from build123d import *

# Parameters (mm, degrees)
F1_DEPTH = 25.4
F0_W     = 244.054224
F0_H     = 73.369068
F2_DEPTH = 23.283333
F3_DEPTH = 4.7625


with BuildPart() as f1:
    # F0 (on Front) → F1 (new body)
    with BuildSketch(Plane.XZ):
        with BuildLine():
            Line((137.143306, 54.800729), (-137.143306, 54.800729))
            ThreePointArc((-137.143306, 54.800729), (-139.264627, 53.922049), (-140.143306, 51.800729))
            Line((-140.143306, 51.800729), (-140.143306, -51.800729))
            ThreePointArc((-140.143306, -51.800729), (-139.264627, -53.922049), (-137.143306, -54.800729))
            Line((-137.143306, -54.800729), (137.143306, -54.800729))
            ThreePointArc((137.143306, -54.800729), (139.264627, -53.922049), (140.143306, -51.800729))
            Line((140.143306, -51.800729), (140.143306, 51.800729))
            ThreePointArc((140.143306, 51.800729), (139.264627, 53.922049), (137.143306, 54.800729))
        make_face()
        with BuildLine():
            ThreePointArc((-127.443306, 39.100729), (-126.564627, 41.222049), (-124.443306, 42.100729))
            Line((-124.443306, 42.100729), (124.443306, 42.100729))
            ThreePointArc((124.443306, 42.100729), (126.564627, 41.222049), (127.443306, 39.100729))
            Line((127.443306, 39.100729), (127.443306, -39.100729))
            ThreePointArc((127.443306, -39.100729), (126.564627, -41.222049), (124.443306, -42.100729))
            Line((124.443306, -42.100729), (-124.443306, -42.100729))
            ThreePointArc((-124.443306, -42.100729), (-126.564627, -41.222049), (-127.443306, -39.100729))
            Line((-127.443306, -39.100729), (-127.443306, 39.100729))
        make_face(mode=Mode.SUBTRACT)
    extrude(amount=F1_DEPTH)

    # F0 (on Front) → F2 (join)
    with BuildSketch(Plane.XZ):
        with BuildLine():
            Line((124.443306, 42.100729), (-124.443306, 42.100729))
            ThreePointArc((-124.443306, 42.100729), (-126.564627, 41.222049), (-127.443306, 39.100729))
            Line((-127.443306, 39.100729), (-127.443306, -39.100729))
            ThreePointArc((-127.443306, -39.100729), (-126.564627, -41.222049), (-124.443306, -42.100729))
            Line((-124.443306, -42.100729), (124.443306, -42.100729))
            ThreePointArc((124.443306, -42.100729), (126.564627, -41.222049), (127.443306, -39.100729))
            Line((127.443306, -39.100729), (127.443306, 39.100729))
            ThreePointArc((127.443306, 39.100729), (126.564627, 41.222049), (124.443306, 42.100729))
        make_face()
        Rectangle(F0_W, F0_H, mode=Mode.SUBTRACT)
    extrude(amount=F2_DEPTH)

    # F0 (on Front) → F3 (join)
    with BuildSketch(Plane.XZ):
        Rectangle(F0_W, F0_H)
    extrude(amount=F3_DEPTH)


solid = f1.part
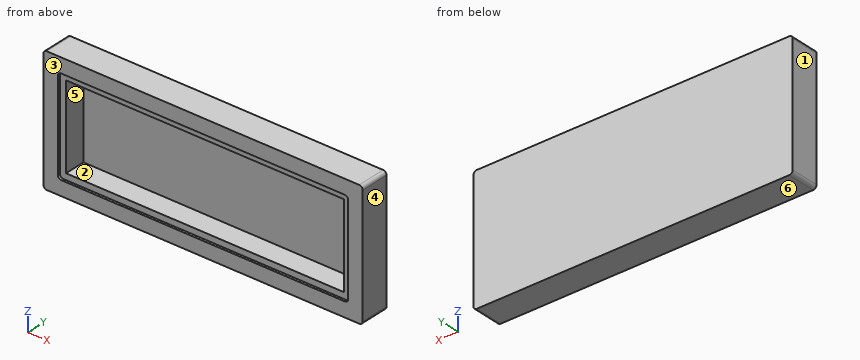
Can you work these out from the model? Positions are in its coordinate system, mm. Face numbers are marked on the shaded views. A direction names the side the tool comes from. Coordinates: 2 decimals unless noted, no trailing zeros. Order: outer loops, then holes, each group sorted by start corner. A loop starts at its lowest first (then second) coordinate and runs counter-clockwise, first axis right, second up. Notation, with made-up numbers: M -23.75,38 L -15.75,38 A10 cw -15.75,52 Z; hole C 18.25,43 d3. An arc over 180 degrees is marked long. Write item = value, one per line.
(1) Suppose I cut it at C-C on x = -75. Please give me the cut outline in (y, z).
Results are:
outline = M -25.4,-54.8 L 0,-54.8 L 0,54.8 L -25.4,54.8 L -25.4,42.1 L -23.28,42.1 L -23.28,36.68 L -4.76,36.68 L -4.76,-36.68 L -23.28,-36.68 L -23.28,-42.1 L -25.4,-42.1 Z
(2) For pin 1 Ø6 at (x, z) = (-104.5, -33) entering from +Y; pin 2 Ø1 at (x, z) = (-97, -16) entering from -Y; pin 3 Ø5 at (x, z) = (63, -35) entering from -Y, each with a flat end and sliding along its axis, tell me the tip position at first contact or that it passes through.
Results are:
pin_1 = 0
pin_2 = -4.76
pin_3 = -23.28
(3) For the marked faces 5 and 6, which set-ups out of +Z, -Z, +X, -X, +Y, -Y let a thin tool reach every point of the face, with its end or its side?
Results are:
face_5 = -Y
face_6 = -Z, +X, -X, +Y, -Y
(4) If we mould it in two halves opening along X, with no side actions, what happens to the marked faces 1, 2, 3 and 4? For each: pulls with the +X half, pulls with the -X half, needs draft (parallel to the pull), parting line crosses it, or undercut.
Results are:
face_1 = pulls with the -X half
face_2 = undercut
face_3 = needs draft
face_4 = pulls with the +X half
(5) Suppose I cut it at B-B on y = -17. Please give me the cut outline in (x, z).
Results are:
outline = M -140.14,-51.8 A3 ccw -137.14,-54.8 L 137.14,-54.8 A3 ccw 140.14,-51.8 L 140.14,51.8 A3 ccw 137.14,54.8 L -137.14,54.8 A3 ccw -140.14,51.8 Z; hole M -122.03,-36.68 L 122.03,-36.68 L 122.03,36.68 L -122.03,36.68 Z
(6) Suppose I cut it at A-A on z = 9. Please give me the cut outline in (x, y).
Results are:
outline = M -140.14,-25.4 L -127.44,-25.4 L -127.44,-23.28 L -122.03,-23.28 L -122.03,-4.76 L 122.03,-4.76 L 122.03,-23.28 L 127.44,-23.28 L 127.44,-25.4 L 140.14,-25.4 L 140.14,0 L -140.14,0 Z
(7) I need wall thicknesses on line 1 along X through (y, z) = (-18.5, 10.5); line 2 along Z through (x, y) = (60.5, -22); line 3 along Z through (x, y) = (-64, -23.5). Which ranges of each line are inside material? Lowest first, please. Write a range as [from, to].
Results are:
line_1 = [-140.14, -122.03], [122.03, 140.14]
line_2 = [-54.8, -36.68], [36.68, 54.8]
line_3 = [-54.8, -42.1], [42.1, 54.8]
